Can you work these out from the model? Positions are in its coordinate system, mm. A direction names the side the tool comes from. Round coordinates to 2 decimals unless told otherwise and drop trailing zeros. Loops run counter-clockwise (first coordinate to the right, second up) from the corner with the lowest first, then second, coordinate; pieces in that order, holes last. Notation, with made-up numbers: (43.5, 53) - (81.5, 53) arc R20 cw to (81.5, 88) - close; hole circle Ø11 at (37.5, 30). An arc over 180 degrees is marked (long way). Answer as CSV lines item,"result".
```python
from build123d import *

# Parameters (mm, degrees)
SKETCH_1_R               = 12.5
SKETCH_1_R_2             = 9.53
EXTRUDE_392_DEPTH        = 7.25
EXTRUDE_595_DEPTH        = 11
CUT_EXTRUDE_875_DEPTH    = 10
HOLE_WIZARD_3_AT_2_COUNT = 2
HOLE_WIZARD_3_AT_2_PITCH = 25
HOLE_WIZARD_3_AT_3_COUNT = 2
HOLE_WIZARD_3_AT_3_PITCH = 35.355339059
HOLE_WIZARD_3_AT_4_COUNT = 2
HOLE_WIZARD_3_AT_4_PITCH = 25
HOLE_WIZARD_1963_D       = 3
EXTRUDE_3682_DEPTH       = 1.6
HOLE_WIZARD_M2_D         = 1.6
HOLE_WIZARD_M2_DEPTH     = 2
HOLE_WIZARD_M2_TIP       = 0.480688495
SKETCH_22_R              = 2.6
CUT_EXTRUDE_4947_DEPTH   = 42.970972112
SKETCH_26_R              = 5.25
EXTRUDE_5417_DEPTH       = 2
CUT_EXTRUDE_5653_DEPTH   = 28.955321497
CHAMFER_1_SIZE           = 1
FILLET_1_R               = 4
CUT_EXTRUDE_6973_DEPTH   = 2.5
HOLE_WIZARD_3_2_D        = 2.5
HOLE_WIZARD_3_2_DEPTH    = 7
HOLE_WIZARD_3_2_TIP      = 0.751075774


with BuildPart() as part:
    # Эскиз1 → Extrude 392 (new body)
    with BuildSketch(Plane(origin=(0, 0, 0), x_dir=(1, 0, 0), z_dir=(0, 1, 0))):
        with Locations(Location((0, 0, 0), (0, 0, 270))):
            Circle(SKETCH_1_R)
        with Locations(Location((0, 0, 0), (0, 0, 270))):
            Circle(SKETCH_1_R_2, mode=Mode.SUBTRACT)
    extrude(amount=-EXTRUDE_392_DEPTH)

    # Эскиз8 → Extrude 595 (add)
    with BuildSketch(Plane.XZ.offset(7.25)):
        with BuildLine():
            Line((-15.5, 17.5), (15.5, 17.5))
            ThreePointArc((15.5, 17.5), (16.914213562, 16.914213562), (17.5, 15.5))
            Line((17.5, 15.5), (17.5, -15.5))
            ThreePointArc((17.5, -15.5), (16.914213562, -16.914213562), (15.5, -17.5))
            Line((15.5, -17.5), (-15.5, -17.5))
            ThreePointArc((-15.5, -17.5), (-16.914213562, -16.914213562), (-17.5, -15.5))
            Line((-17.5, -15.5), (-17.5, 15.5))
            ThreePointArc((-17.5, 15.5), (-16.914213562, 16.914213562), (-15.5, 17.5))
        make_face()
    extrude(amount=EXTRUDE_595_DEPTH)

    # Эскиз9 → Cut-Extrude 875 (cut)
    with BuildSketch(Plane.XZ.offset(18.25)):
        with BuildLine():
            Line((-6.5, 16), (6.5, 16))
            ThreePointArc((6.5, 16), (7.914213562, 15.414213562), (8.5, 14))
            Line((8.5, 14), (8.5, -14))
            ThreePointArc((8.5, -14), (7.914213562, -15.414213562), (6.5, -16))
            Line((6.5, -16), (-6.5, -16))
            ThreePointArc((-6.5, -16), (-7.914213562, -15.414213562), (-8.5, -14))
            Line((-8.5, -14), (-8.5, 14))
            ThreePointArc((-8.5, 14), (-7.914213562, 15.414213562), (-6.5, 16))
        make_face()
    extrude(amount=-CUT_EXTRUDE_875_DEPTH, mode=Mode.SUBTRACT)

    # Эскиз10 → Hole Wizard 3 (revolve, cut)
    with BuildSketch(Plane(origin=(-12.5, -7.25, -12.5), x_dir=(0, 0, 1), z_dir=(1, 0, 0))):
        Polygon((0, 0), (0, 11), (1.7, 11), (1.7, 3.425), (1.725, 3.4), (3.25, 3.4), (3.25, 0), align=None)
    hole_wizard_3 = revolve(axis=Axis((-12.5, -0.9, -12.5), (0, -1, 0)), mode=Mode.SUBTRACT)

    # Hole Wizard 3 at 2: Hole Wizard 3 ×2
    with Locations(*[(i * HOLE_WIZARD_3_AT_2_PITCH, 0, 0) for i in range(1, HOLE_WIZARD_3_AT_2_COUNT)]):
        add(hole_wizard_3, mode=Mode.SUBTRACT)

    # Hole Wizard 3 at 3: Hole Wizard 3 ×2
    with Locations(*[Vector(0.7071067811865476, 0, 0.7071067811865476) * (i * HOLE_WIZARD_3_AT_3_PITCH) for i in range(1, HOLE_WIZARD_3_AT_3_COUNT)]):
        add(hole_wizard_3, mode=Mode.SUBTRACT)

    # Hole Wizard 3 at 4: Hole Wizard 3 ×2
    with Locations(*[(0, 0, i * HOLE_WIZARD_3_AT_4_PITCH) for i in range(1, HOLE_WIZARD_3_AT_4_COUNT)]):
        add(hole_wizard_3, mode=Mode.SUBTRACT)

    # Hole Wizard 1963 (through all)
    with Locations(Plane(origin=(0, -7.25, 0), x_dir=(1, 0, 0), z_dir=(0, 1, 0))):
        with Locations((0, -14.3), (-5, -14.3), (5, -14.3)):
            Hole(HOLE_WIZARD_1963_D / 2)

    # Эскиз29 → Extrude 3682 (add)
    with BuildSketch(Plane.XZ.offset(8.25)):
        with BuildLine():
            Line((-6.5, -5), (-8.5, -5))
            Line((-8.5, -5), (-8.5, -8))
            Line((-8.5, -8), (-6.5, -8))
            ThreePointArc((-6.5, -8), (-5, -6.5), (-6.5, -5))
        make_face()
        with BuildLine():
            Line((6.5, -5), (8.5, -5))
            Line((8.5, -5), (8.5, -8))
            Line((8.5, -8), (6.5, -8))
            ThreePointArc((6.5, -8), (5, -6.5), (6.5, -5))
        make_face()
        with BuildLine():
            Line((-6.5, 8), (-8.5, 8))
            Line((-8.5, 8), (-8.5, 5))
            Line((-8.5, 5), (-6.5, 5))
            ThreePointArc((-6.5, 5), (-5, 6.5), (-6.5, 8))
        make_face()
        with BuildLine():
            Line((6.5, 8), (8.5, 8))
            Line((8.5, 8), (8.5, 5))
            Line((8.5, 5), (6.5, 5))
            ThreePointArc((6.5, 5), (5, 6.5), (6.5, 8))
        make_face()
    extrude(amount=EXTRUDE_3682_DEPTH)

    # Крепление платы M2
    with Locations(Plane(origin=(0, -9.85, 0), x_dir=(-1, 0, 0), z_dir=(0, -1, 0))):
        with Locations((6.5, -6.5), (-6.5, -6.5), (6.5, 6.5), (-6.5, 6.5)):
            Hole(HOLE_WIZARD_M2_D / 2, depth=HOLE_WIZARD_M2_DEPTH)
            with Locations((0, 0, -(HOLE_WIZARD_M2_DEPTH + HOLE_WIZARD_M2_TIP / 2))):  # 118° drill point
                Cone(0, HOLE_WIZARD_M2_D / 2, HOLE_WIZARD_M2_TIP, mode=Mode.SUBTRACT)

    # Эскиз22 → Cut-Extrude 4947 (cut, through all)
    with BuildSketch(Plane(origin=(0, 0, -16), x_dir=(-1, 0, 0), z_dir=(0, 0, -1))):
        with Locations((0, -13.95)):
            Circle(SKETCH_22_R)
    extrude(amount=CUT_EXTRUDE_4947_DEPTH, mode=Mode.SUBTRACT)

    # Эскиз26 → Extrude 5417 (add)
    with BuildSketch(Plane(origin=(0, -7.25, 0), x_dir=(1, 0, 0), z_dir=(0, 1, 0))):
        with Locations(Location((0, 0, 0), (0, 0, 90))):
            Circle(SKETCH_26_R)
    extrude(amount=EXTRUDE_5417_DEPTH)

    # Эскиз25 → Cut-Extrude 5653 (cut, through all)
    with BuildSketch(Plane(origin=(0, -5.25, 0), x_dir=(1, 0, 0), z_dir=(0, 1, 0))):
        with BuildLine():
            Line((-1.21, 3.21), (1.21, 3.21))
            ThreePointArc((1.21, 3.21), (2.624213562, 2.624213562), (3.21, 1.21))
            Line((3.21, 1.21), (3.21, -1.21))
            ThreePointArc((3.21, -1.21), (2.624213562, -2.624213562), (1.21, -3.21))
            Line((1.21, -3.21), (-1.21, -3.21))
            ThreePointArc((-1.21, -3.21), (-2.624213562, -2.624213562), (-3.21, -1.21))
            Line((-3.21, -1.21), (-3.21, 1.21))
            ThreePointArc((-3.21, 1.21), (-2.624213562, 2.624213562), (-1.21, 3.21))
        make_face()
    extrude(amount=-CUT_EXTRUDE_5653_DEPTH, mode=Mode.SUBTRACT)

    # Фаска 1
    chamfer_1_edges = [part.edges().sort_by_distance(p)[0] for p in [
        (0, -7.25, -17.5),
        (16.914213562, -7.25, -16.914213562),
        (17.5, -7.25, 0),
        (16.914213562, -7.25, 16.914213562),
        (0, -7.25, 17.5),
        (-16.914213562, -7.25, 16.914213562),
        (-17.5, -7.25, 0),
        (0, 0, -12.5),
        (-16.914213562, -7.25, -16.914213562),
    ]]
    chamfer(chamfer_1_edges, length=CHAMFER_1_SIZE)

    # Скругление1
    # the kernel refuses this fillet: 4 mm, written as the material it adds along each edge
    with BuildSketch(Plane(origin=(8.5, -8.25, -8), x_dir=(0, 0, -1), z_dir=(0, -1, 0)), Plane(origin=(8.5, -8.25, 5), x_dir=(0, 0, -1), z_dir=(0, -1, 0)), Plane(origin=(-8.5, -8.25, 8), x_dir=(0, 0, 1), z_dir=(0, -1, 0)), Plane(origin=(-8.5, -8.25, -5), x_dir=(0, 0, 1), z_dir=(0, -1, 0))) as fillet_1_piece_1:
        with BuildLine():
            CenterArc((3.623475383, -4), FILLET_1_R, 90, 68.676313736)
            Line((-0.102688532, -2.545454545), (-0.475304923, -2.4))
            ThreePointArc((-0.475304923, -2.4), (-0.4, -2), (-0.4, 0))
            Line((-0.4, 0), (0, 0.4))
            Line((0, 0.4), (3.623475383, 0.4))
            Line((3.623475383, 0.4), (3.623475383, 0))
        make_face()
    extrude(amount=1.6)
    with BuildSketch(Plane(origin=(8.5, -8.25, -5), x_dir=(0, 0, 1), z_dir=(0, -1, 0)), Plane(origin=(8.5, -8.25, 8), x_dir=(0, 0, 1), z_dir=(0, -1, 0)), Plane(origin=(-8.5, -8.25, 5), x_dir=(0, 0, -1), z_dir=(0, -1, 0)), Plane(origin=(-8.5, -8.25, -8), x_dir=(0, 0, -1), z_dir=(0, -1, 0))) as fillet_1_piece_2:
        with BuildLine():
            CenterArc((3.623475383, 4), FILLET_1_R, 201.323686264, 68.676313736)
            Line((-0.102688532, 2.545454545), (-0.475304923, 2.4))
            ThreePointArc((-0.475304923, 2.4), (-0.4, 2), (-0.4, 0))
            Line((-0.4, 0), (0, -0.4))
            Line((0, -0.4), (3.623475383, -0.4))
            Line((3.623475383, -0.4), (3.623475383, 0))
        make_face()
    extrude(amount=1.6)

    # Эскиз36 → Cut-Extrude 6973 (cut)
    with BuildSketch(Plane.XZ.offset(18.25)):
        with BuildLine():
            Line((-14, 16), (14, 16))
            ThreePointArc((14, 16), (15.414213562, 15.414213562), (16, 14))
            Line((16, 14), (16, -14))
            ThreePointArc((16, -14), (15.414213562, -15.414213562), (14, -16))
            Line((14, -16), (-14, -16))
            ThreePointArc((-14, -16), (-15.414213562, -15.414213562), (-16, -14))
            Line((-16, -14), (-16, 14))
            ThreePointArc((-16, 14), (-15.414213562, 15.414213562), (-14, 16))
        make_face()
    extrude(amount=-CUT_EXTRUDE_6973_DEPTH, mode=Mode.SUBTRACT)

    # Hole Wizard 3 2
    with Locations(Plane(origin=(0, -15.75, 0), x_dir=(-1, 0, 0), z_dir=(0, -1, 0))):
        with Locations((11.75, 0), (-11.75, 0)):
            Hole(HOLE_WIZARD_3_2_D / 2, depth=HOLE_WIZARD_3_2_DEPTH)
            with Locations((0, 0, -(HOLE_WIZARD_3_2_DEPTH + HOLE_WIZARD_3_2_TIP / 2))):  # 118° drill point
                Cone(0, HOLE_WIZARD_3_2_D / 2, HOLE_WIZARD_3_2_TIP, mode=Mode.SUBTRACT)


solid = part.part
```
Q1. Imagine slicing it at A-A (y = -13.95). Write out the boundary of the cut face in (x, z).
Checks:
outline,"(-17.5, -15.5) arc R2 ccw to (-15.5, -17.5) - (-2.6, -17.5) - (-2.6, -16) - (-6.5, -16) arc R2 cw to (-8.5, -14) - (-8.5, 14) arc R2 cw to (-6.5, 16) - (6.5, 16) arc R2 cw to (8.5, 14) - (8.5, -14) arc R2 cw to (6.5, -16) - (2.6, -16) - (2.6, -17.5) - (15.5, -17.5) arc R2 ccw to (17.5, -15.5) - (17.5, 15.5) arc R2 ccw to (15.5, 17.5) - (-15.5, 17.5) arc R2 ccw to (-17.5, 15.5) - close; hole circle Ø3.4 at (-12.5, -12.5); hole circle Ø3.4 at (-12.5, 12.5); hole circle Ø2.5 at (-11.75, 0); hole circle Ø2.5 at (11.75, 0); hole circle Ø3.4 at (12.5, -12.5); hole circle Ø3.4 at (12.5, 12.5)"
Q2. If I drill on line 1 along Z through (x, y) = (-12.5, -8.3); line 2 along X through (y, z) = (-13, -10.5); line 3 along Z through (x, y) = (0, -7.6), over which ranges is the centre line in solid material (lowest first)? Write a range as [from, to].
Checks:
line 1,"[-17.5, -15.75], [-9.25, 9.25], [15.75, 17.5]"
line 2,"[-17.5, -8.5], [8.5, 17.5]"
line 3,"[-16.85, -3.21], [3.21, 12.8], [15.8, 16.85]"
Q3. Imagine slicing it at C-C (y = -4.25). Write out the boundary of the cut face in (x, z), then the cut area to 3 significant figures.
Checks:
outline,"circle Ø25 at (0, 0); hole circle Ø19.06 at (0, 0)"
area,"206 mm²"
Q4. We'd pull the mould along Z, two halves only. Please class faces 5 (the flat face through (-17.01, -7.76, -0.22)), 6 (the cylindrical face through (-15.43, -17.02, 15.4)), 7 (the flat face through (0, -11, -17.5)): pulls with the +Z half, pulls with the -Z half, needs draft (parallel to the pull), parting line crosses it, or undercut.
Checks:
face 5,"needs draft"
face 6,"undercut"
face 7,"pulls with the -Z half"
Q5. Imagine slicing it at B-B (x = 0). Count the separate pieces of the cut face and the enclosed holes in it, then the cut area to 3 significant figures.
Checks:
separate pieces,"4"
enclosed holes,"0"
area,"97.0 mm²"
Q6. On a 3-axis mill with a long thin cutter (end or side, diameter ignored), from which of +Z, -Z, +X, -X, +Y, -Y can I reach the whole of each face in a straight line? I mean faces 1 (the cylindrical face through (11.52, -8.93, 15.6)), 2 (the flat face through (9, 0, -4)), 3 (the flat face through (16, -17, 0)), 4 (the flat face through (0, -7, -3.21)). Say none if no direction works.
Checks:
face 1,"+Y"
face 2,"+Z, -Z, +X, -X, +Y"
face 3,"-Y"
face 4,"+Y, -Y"
Q7. I'm going to push flat-ended pins straight in: pin 1 Ø0.7 at (x, y) = (-0.5, -7.5) entering from -Z; pin 2 Ø1.5 at (x, z) = (11.75, 0) entering from -Y; pin 3 Ø6 at (x, z) = (-12.5, -12.5) entering from -Y; pin 4 Ø21 at (x, z) = (3, 1.5) entering from +Y. Where does each tip first touch, or does it pass through?
Checks:
pin 1,"z = -17.1"
pin 2,"y = -8.45"
pin 3,"y = -15.75"
pin 4,"y = 0"
